Check sheet for the drawn part. Datum: minimum x, y, z corner. Units: mm. Coordinates: 2 decimals unless noted, no trailing zeros. Order: outer loops, then holes, each group sorted by start corner. A loop starts at its lowest first (then second) coordinate and runs counter-clockwise, first axis right, second up. Notation, with made-up numbers: M 60,-40 L 94,-40 A20 ccw 94,-27 Z; hole C -35,-3.5 d2. An arc over 180 degrees is marked long. Return JSON: item names as keys, results as strings. Group by question number.
Q1. Section check D-D, the plane z = 22. Enter the section's corners in (x, y).
Q2. Section check B-B, the plane x = 98.5. Enter the section's corners in (y, z) (3 decimals), then the cut area to 3 significant figures.
Q3. Section check C-C, the plane x = 54. Enter the section's corners in (y, z) (3 decimals).
Q4. Go/stop test with flat-tipped pins: pin 1 Ø6.5 at (y, z) = (72, 45) entering from +X; pin 2 Ø10 at (x, y) = (88.5, 19.5) entering from +Z; pin 3 Ø8 at (x, z) = (54, 14) entering from -Y; pin 4 Ø5 at (y, z) = (68, 49) entering from +X (1 decimal). Record where each tip stops, or that it passes through.
Q5. Section check A-A, the plane y = 71. Enter the section's corners in (x, z) (3 decimals).
Q6. Thickness scan on probe 1 along Z at (x, y) = (198, 17) (1 decimal); probe 2 along Z at (x, y) = (111.5, 95); probe 3 along X at (y, z) = (17.5, 23). Record the ranges inside material, lowest first.
Q7. Mould release check, pull along X, two halves, no side actions. Record for the marked faces 1, 2 and 3: pulls with the +X half, pulls with the -X half, needs draft (parallel to the pull), parting line crosses it, or undercut.
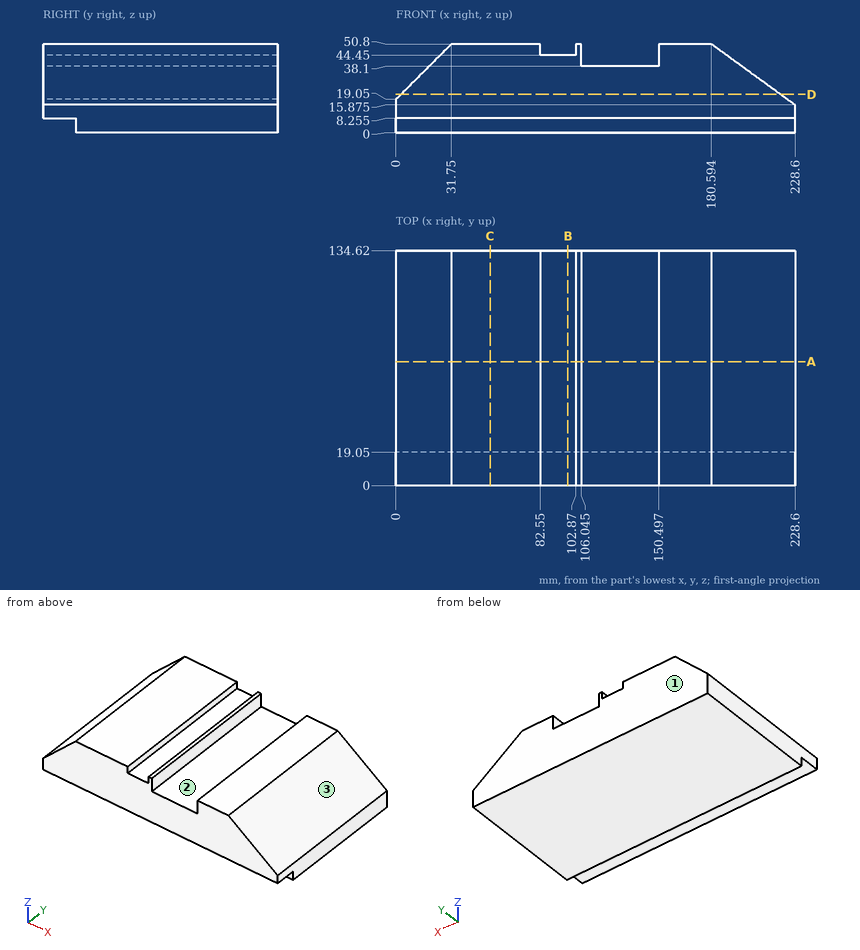
Numbers:
{
 "1": {"outline": "M 2.95,0 L 220.18,0 L 220.18,134.62 L 2.95,134.62 Z"},
 "2": {"outline": "M 0,8.255 L 19.05,8.255 L 19.05,0 L 134.62,0 L 134.62,44.45 L 0,44.45 Z", "area": "5,830 mm2"},
 "3": {"outline": "M 0,8.255 L 19.05,8.255 L 19.05,0 L 134.62,0 L 134.62,50.8 L 0,50.8 Z"},
 "4": {"pin 1": "stops at x = 193.03", "pin 2": "stops at z = 44.45", "pin 3": "stops at y = 0", "pin 4": "stops at x = 186.5"},
 "5": {"outline": "M 0,0 L 228.6,0 L 228.6,15.875 L 180.594,50.8 L 150.497,50.8 L 150.497,38.1 L 106.045,38.1 L 106.045,50.8 L 102.87,50.8 L 102.87,44.45 L 82.55,44.45 L 82.55,50.8 L 31.75,50.8 L 0,19.05 Z"},
 "6": {"probe 1": "z = 8.3 to 38.1", "probe 2": "z = 0 to 38.1", "probe 3": "x = 3.95 to 218.81"},
 "7": {"face 1": "needs draft", "face 2": "undercut", "face 3": "pulls with the +X half"}
}
